Can you work these out from the drawing? Everything is in mm from the part's minimum corner. A direction names the side the tool comes from. Give positions to 0.01 mm unless a question says otherwise; leave off trailing zeros. Write each loop counter-clockwise with the first axis right and the second up, starting at its lowest first coordinate (ties: lowest second). Pieces come first, ordered by that corner, then holes. Notation, with made-up numbers: (83, -15.75) - (112, -15.75) arc R20 cw to (112, -2.75) - close; hole circle Ø10 at (27.5, -14). An arc over 180 degrees is marked (long way). Use a Markdown table: item, result. Add a question column.
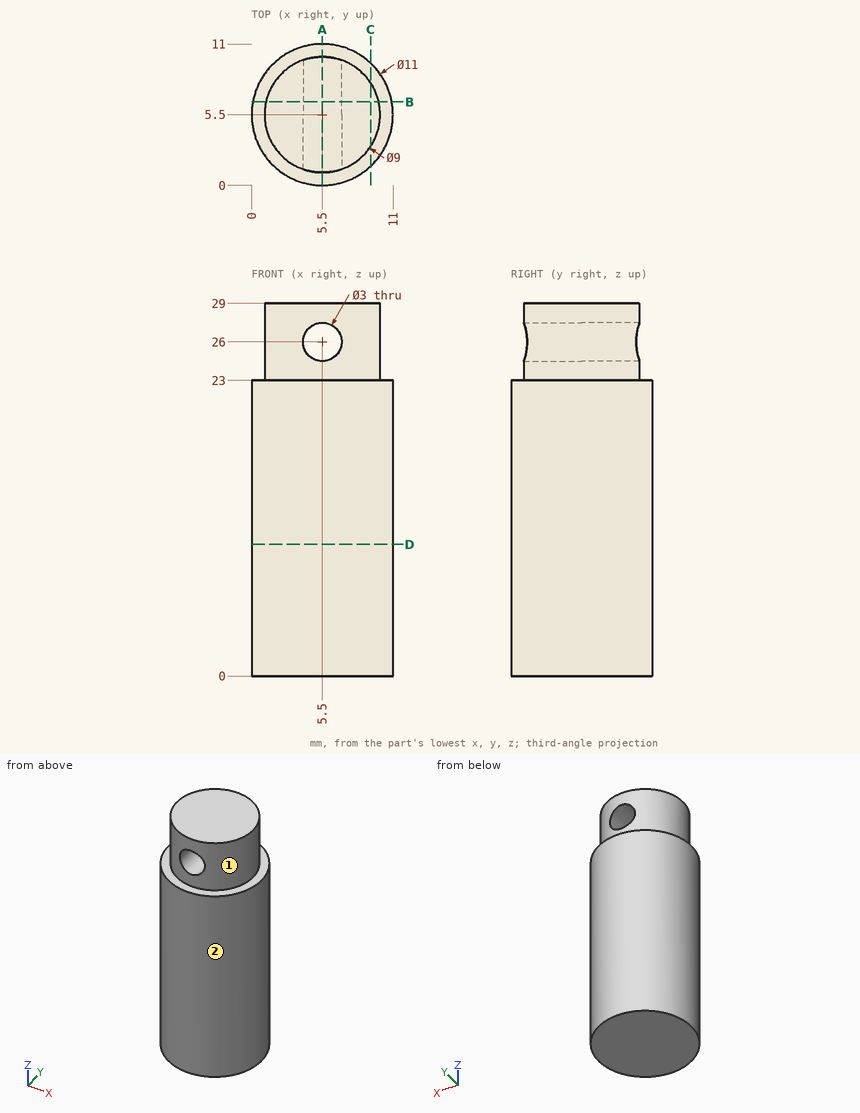
Q1. If I drill on probe 1 along Z at (x, y) = (5.5, 6.4); probe 2 along Z at (x, y) = (5, 5.5); probe 3 along X at (y, z) = (4.2, 26), over which ranges is the centre line in solid material (lowest first)? Write a range as [from, to].
Q2. On a 3-axis mill with a long thin cutter (end or side, diameter ignored), from which of +Z, -Z, +X, -X, +Y, -Y can I reach the whole of each face in a straight line? I mean the marked faces 1 and 2. Say none if no direction works.
Q3. Suppose I cut it at A-A (x = 5.5). Please give me the cut outline in (y, z).
Q4. I'm going to push flat-ended pins straight in: P1, Ø3, axis at x = 9, z = 13, coming from the +Y side; P2, Ø1.5, axis at x = 2, z = 20.5, coming from the -Y side; P3, Ø1.5, axis at y = 4.5, z = 12, coming from the +X side. Where does each tip first touch, or does it pass through?
Q5. Suppose I cut it at C-C (x = 9.25). Please give me the cut outline in (y, z).
Q6. Suppose I cut it at D-D (z = 10.25). Please give me the cut outline in (x, y).
Q7. Suppose I cut it at B-B (y = 6.5). Please give me the cut outline in (x, z), and give its area (3 significant figures).
Derived:
| question | item | result |
|---|---|---|
| 1 | probe 1 | [0, 24.5], [27.5, 29] |
| 1 | probe 2 | [0, 24.59], [27.41, 29] |
| 1 | probe 3 | [1.19, 4], [7, 9.81] |
| 2 | face 1 | +Z |
| 2 | face 2 | +Z, -Z |
| 3 | outline | (0, 0) - (11, 0) - (11, 23) - (10, 23) - (10, 24.5) - (1, 24.5) - (1, 23) - (0, 23) - close; (1, 27.5) - (10, 27.5) - (10, 29) - (1, 29) - close |
| 4 | P1 | y = 10.62 |
| 4 | P2 | y = 0.74 |
| 4 | P3 | x = 10.99 |
| 5 | outline | (1.48, 0) - (9.52, 0) - (9.52, 23) - (7.99, 23) - (7.99, 29) - (3.01, 29) - (3.01, 23) - (1.48, 23) - close |
| 6 | outline | circle Ø11 at (5.5, 5.5) |
| 7 | outline | (0.09, 0) - (10.91, 0) - (10.91, 23) - (9.89, 23) - (9.89, 29) - (1.11, 29) - (1.11, 23) - (0.09, 23) - close; hole circle Ø3 at (5.5, 26) |
| 7 | area | 294 mm² |
